The model under review builds one solid part; all positions refer to its coordinate system, in mm. A direction names the side the tool comes from. Round coordinates to 2 decimals unless told otherwise and drop trailing zeros. Order: outer loops, then holes, each group sorted by start corner. A loop starts at its lowest first (then second) coordinate and runs counter-clockwise, first axis right, second up.
1) Mouldability with a two-part tool opening along Z and no side actions: class faces 1 (the face through (2, 0, 1)), 2 (the face through (1.341, 4.93, -3.233)), 3 (the face through (1.103, 6.119, 0.245)) as pulls with the +Z half, pulls with the -Z half, needs draft (parallel to the pull), parting line crosses it, or undercut.
2) Machinability: for faces 4 (the face through (2, 12.4, 0)), 5 (the face through (2, 10, -2)), which of the approach directions +Z, -Z, +X, -X, +Y, -Y give a long, thin tool a straight path to every point of the face, cutting with its end or side? Answer none if there is none.
3) Consider section D-D (z = -2). Give the boundary of the cut face in (x, y).
4) Consider section B-B (z = 0). Give the boundary of the cut face in (x, y).
5) Clearance check with flat-ended pins moving along their axes: P1, Ø1.5, axis at y = 10.5, z = 1, coming from the -X side; P2, Ø1, axis at x = -2, y = 7.5, coming from the -Z side; P3, Ø3, axis at y = 2.5, z = 2, coming from the +X side. State where each tip first meets the part, or that it passes through.
6) Consider section A-A (x = 0). Give the boundary of the cut face in (y, z).
7) To check wall thickness, follow L1, parallel to X at y = 3.75, z = 0; L2, parallel to X at y = 6, z = 0.5. State the ranges of each line that lie inside material, in increasing order.
8) Consider section C-C (y = 9). Give the boundary of the cut face in (x, z).
from build123d import *


with BuildPart() as part:
    # Эскиз1 → Повернуть1 (revolve)
    with BuildSketch(Plane(origin=(0, 0, 0), x_dir=(0, 0, -1), z_dir=(1, 0, 0))):
        Polygon((0, 0), (0, 12.4), (2.2, 12.4), (2.2, 10), (3.5, 10), (3.5, 0), align=None)
    revolve(axis=Axis((0, 0, 0), (0, 1, 0)))

    # Эскиз2 → Отверстие обработанное метчиком #4-401 (revolve, cut)
    with BuildSketch(Plane(origin=(0, 0, 0), x_dir=(0, 0, -1), z_dir=(1, 0, 0))):
        Polygon((0, 0), (0, 12.4), (1.6764, 12.4), (1.1303, 12.017616663), (1.1303, 0.382383337), (1.6764, 0), align=None)
    revolve(axis=Axis((0, -6.35, 0), (0, 1, 0)), mode=Mode.SUBTRACT)


solid = part.part
Answer below:
1. face 1: needs draft
1. face 2: parting line crosses it
1. face 3: undercut
2. face 4: +Z, -Z, +X, -X, +Y
2. face 5: +Y
3. outline: (-2.87, 0) - (2.87, 0) - (2.87, 10) - (0.92, 10) - (0.92, 12.4) - (-0.92, 12.4) - (-0.92, 10) - (-2.87, 10) - close
4. outline: (-3.5, 0) - (-1.68, 0) - (-1.13, 0.38) - (-1.13, 12.02) - (-1.68, 12.4) - (-2.2, 12.4) - (-2.2, 10) - (-3.5, 10) - close; (1.13, 0.38) - (1.68, 0) - (3.5, 0) - (3.5, 10) - (2.2, 10) - (2.2, 12.4) - (1.68, 12.4) - (1.13, 12.02) - close
5. P1: stops at x = -3.47
5. P2: stops at z = -3.16
5. P3: stops at x = 3.46
6. outline: (0, -3.5) - (10, -3.5) - (10, -2.2) - (12.4, -2.2) - (12.4, -1.68) - (12.02, -1.13) - (0.38, -1.13) - (0, -1.68) - close; (0, 1.68) - (0.38, 1.13) - (12.02, 1.13) - (12.4, 1.68) - (12.4, 2.2) - (10, 2.2) - (10, 3.5) - (0, 3.5) - close
7. L1: x = -3.5 to -1.13, 1.13 to 3.5
7. L2: x = -3.46 to -1.01, 1.01 to 3.46
8. outline: circle Ø7 at (0, 0); hole circle Ø2.26 at (0, 0)
